Verification items for this drawing (mm, ordinates from the low corner). A direction names the side the tool comes from. Round coordinates to 2 decimals unless told otherwise and drop trailing zeros. Write each loop counter-clockwise with the first axis right and the second up, starting at its lowest first coordinate (ties: lowest second). Pieces come first, ordered by that corner, then holes.
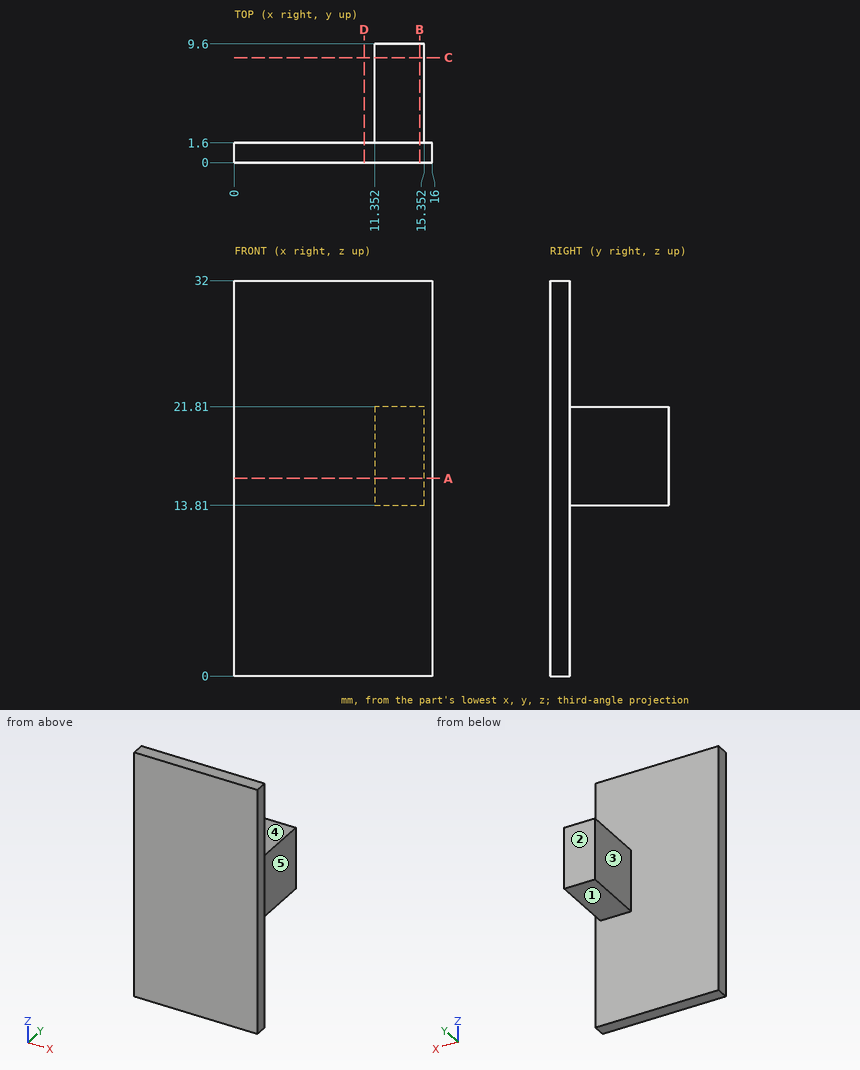
1. Access from +Z, -Z, +X, -X, +Y, -Y to the whole of each face (thin tool, end or side, straight path). Record for the marked faces 1, 2, 3, 4 and 5.
2. Section check A-A (z = 16). Record the cut outline in (x, y).
3. Scan lines: line 1 along Z through (x, y) = (12, 6); line 2 along Y through (x, z) = (1.75, 22); line 3 along X through (y, z) = (9.25, 16.5). Record each from-to range of solid material in increasing order.
4. Section check C-C (y = 8.5). Record the cut outline in (x, z), plus the area to 3 significant figures.
5. Depth check by flat-ended pin: pin 1 Ø1.2 at (x, y) = (14, 4.5) entering from -Z; pin 2 Ø2.5 at (y, z) = (5, 18.5) entering from -X; pin 3 Ø5 at (x, z) = (4, 19) entering from +Y. Enter the tip coordinate at first touch or a pass-through.
6. Section check B-B (x = 15). Record the cut outline in (y, z), plus the area to 3 significant figures.
7. Section check D-D (x = 10.5). Record the cut outline in (y, z).
Results below:
1. face 1: -Z, +X, -X, +Y
1. face 2: +Z, -Z, +X, -X, +Y
1. face 3: +Z, -Z, -X, +Y
1. face 4: +Z, +X, -X, +Y
1. face 5: +Z, -Z, +X, +Y
2. outline: (0, 0) - (16, 0) - (16, 1.6) - (15.35, 1.6) - (15.35, 9.6) - (11.35, 9.6) - (11.35, 1.6) - (0, 1.6) - close
3. line 1: z = 13.81 to 21.81
3. line 2: y = 0 to 1.6
3. line 3: x = 11.35 to 15.35
4. outline: (11.35, 13.81) - (15.35, 13.81) - (15.35, 21.81) - (11.35, 21.81) - close
4. area: 32.0 mm2
5. pin 1: stops at z = 13.81
5. pin 2: stops at x = 11.35
5. pin 3: stops at y = 1.6
6. outline: (0, 0) - (1.6, 0) - (1.6, 13.81) - (9.6, 13.81) - (9.6, 21.81) - (1.6, 21.81) - (1.6, 32) - (0, 32) - close
6. area: 115 mm2
7. outline: (0, 0) - (1.6, 0) - (1.6, 32) - (0, 32) - close
